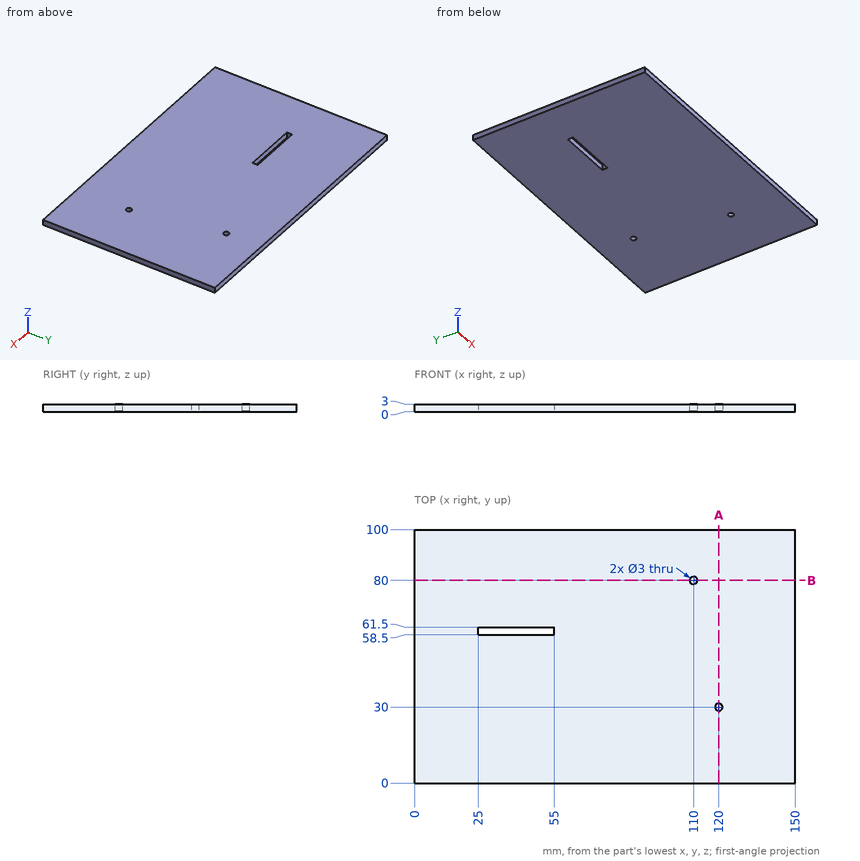
For this review, use the dimensioned drawing (mm, ordinates from the lowest corner) and the shaded views. Give positions to 0.01 mm unless a question says otherwise; leave off trailing zeros. Loops run counter-clockwise (first coordinate to the right, second up) from the corner with the lowest first, then second, coordinate; pieces in that order, holes last. Notation, with made-up numbers: (79.5, 11) - (93.5, 11) arc R13 ccw to (93.5, 17) - close; hole circle Ø5 at (-15.75, -25). An arc over 180 degrees is marked (long way). Write each question's results on one line, items separated by ' | '.
(1) For pin 1 Ø1.8 at (x, y) = (120, 30) entering from -Z, flat-tipped, find the tip position at first contact; note if it passes through.
Conclusion:
pin 1: through
(2) Take a section at B-B (y = 80). Give the boundary of the cut face in (x, z), then the cut area to 3 significant figures.
Conclusion:
outline: (0, 0) - (108.5, 0) - (108.5, 3) - (0, 3) - close; (111.5, 0) - (150, 0) - (150, 3) - (111.5, 3) - close | area: 441 mm^2
(3) Take a section at A-A (x = 120). Give the boundary of the cut face in (y, z), then the cut area to 3 significant figures.
Conclusion:
outline: (0, 0) - (28.5, 0) - (28.5, 3) - (0, 3) - close; (31.5, 0) - (100, 0) - (100, 3) - (31.5, 3) - close | area: 291 mm^2
(4) For line 1 along Y through (x, z) = (110, 1.4); line 2 along Y through (x, z) = (120, 1.95); line 3 along X through (y, z) = (79, 0.7), list the stretches that pass through material, from the lowest coordinate up.
Conclusion:
line 1: 0 to 78.5, 81.5 to 100 | line 2: 0 to 28.5, 31.5 to 100 | line 3: 0 to 108.88, 111.12 to 150
